from build123d import *

# Parameters (mm, degrees)
FILLET_4_R      = 3
F_4_0MM_4_D     = 4
F_4_0MM_4_DEPTH = 8
F_4_0MM_4_TIP   = 1.201721238
F_4_0MM_5_D     = 4
F_4_0MM_5_DEPTH = 7
F_4_0MM_5_TIP   = 1.201721238


# Read off the part's stored shape, not the designer's step: M16 机械螺纹 螺柱1
with BuildPart() as part:
    # 草图1 → 旋转1 (revolve)
    with BuildSketch(Plane.XY, mode=Mode.PRIVATE) as revolve_1_sk:
        Polygon((0, 0), (0, 8), (27, 8), (27, 8.5), (83, 8.5), (83, 18), (65, 18), (65, 27), (113, 27), (113, 18), (95, 18), (95, 8.5), (140, 8.5), (140, 0), align=None)
    revolve(revolve_1_sk.sketch.rotate(Axis((0, 0, 0), (1, 0, 0)), 90), axis=Axis((0, 0, 0), (1, 0, 0)))

    # 圆角4
    fillet_4_edges = [part.edges().sort_by_distance(p)[0] for p in [
        (95, 0, -8.5),
        (95, 0, -18),
        (83, 0, -18),
        (83, 0, -8.5),
    ]]
    fillet(fillet_4_edges, radius=FILLET_4_R)

    # M16 机械螺纹 螺柱1 outline → M16 机械螺纹 螺柱1 (revolve, cut)
    with BuildSketch(Plane.YX):
        Polygon((8, 1.0825), (6.9175, 0), (8, 0), align=None)
    revolve(axis=Axis((0, 0, 0), (1, 0, 0)), mode=Mode.SUBTRACT)

    # Ø4.0mm 暗销孔4
    with Locations(Plane(origin=(17.1, 8, 0), x_dir=(0, 0, 1), z_dir=(0, 1, 0))):
        with Locations((0, 0)):
            Hole(F_4_0MM_4_D / 2, depth=F_4_0MM_4_DEPTH)
            with Locations((0, 0, -(F_4_0MM_4_DEPTH + F_4_0MM_4_TIP / 2))):  # 118° drill point
                Cone(0, F_4_0MM_4_D / 2, F_4_0MM_4_TIP, mode=Mode.SUBTRACT)

    # Ø4.0mm 暗销孔5
    with Locations(Plane(origin=(140, 0, 0), x_dir=(0, 0, -1), z_dir=(1, 0, 0))):
        with Locations((0, 0)):
            Hole(F_4_0MM_5_D / 2, depth=F_4_0MM_5_DEPTH)
            with Locations((0, 0, -(F_4_0MM_5_DEPTH + F_4_0MM_5_TIP / 2))):  # 118° drill point
                Cone(0, F_4_0MM_5_D / 2, F_4_0MM_5_TIP, mode=Mode.SUBTRACT)


solid = part.part
Here's how the part is built. I have some questions about the finished solid (model axes, mm). A direction names the side the tool comes from. Coordinates: 2 decimals unless noted, no trailing zeros. Write each loop counter-clockwise with the first axis right and the second up, starting at its lowest first coordinate (ties: lowest second). Pieces come first, ordered by that corner, then holes.
1) If we section it at D-D (y = 21): List the corners of the cut face in (x, z) for me.
Filled in:
outline: (65, -16.97) - (113, -16.97) - (113, 16.97) - (65, 16.97) - close
2) Thinking about a two-plate mould opening in Y: for faces 4 (the face through (119.294, -8.428, -1.107)), 5 (the face through (89.34, 26.36, -5.85)), 6 (the face through (15.148, 3.948, 0.434)), 7 (the face through (17.204, -0.993, 0.331)), which applies, +Y half, -Y half, draft (parallel to the pull), parting line (faces both ways), or undercut?
Filled in:
face 4: undercut
face 5: parting line
face 6: draft
face 7: +Y half
3) I'm going to push flat-ended pins straight in: pin 1 (12 mm diameter, centred on y = -3.5, z = -17.5, fed in from -X); pin 2 (8 mm diameter, centred on x = 91, z = -15.5, fed in from +Y); pin 3 (13.5 mm diameter, centred on y = 1.5, z = -3, fed in from -X); pin 4 (3 mm diameter, centred on y = 7.5, z = -13.5, fed in from -X). Where does each tip first touch, or does it pass through?
Filled in:
pin 1: stops at x = 65
pin 2: stops at y = 24.43
pin 3: stops at x = 0
pin 4: stops at x = 82.29
4) If we section it at A-A (x = 102): List the corners of the cut face in (y, z) for me, plus the area to 3 significant figures.
Filled in:
outline: circle Ø54 at (0, 0); circle Ø17 at (0, 0); hole circle Ø36 at (0, 0)
area: 1,500 mm2
5) Which directions (+Z, -Z, +X, -X, +Y, -Y) give clear straight access to the entire face, cutting with the end or side of a thin tool? Please do faces 1 (the face through (113, 18, 6)), 2 (the face through (0, 0, 0)), 3 (the face through (72.395, -12.165, -13.267)).
Filled in:
face 1: +X
face 2: +Z, -Z, -X, +Y, -Y
face 3: -X
6) If we section it at C-C (z = -23): List the corners of the cut face in (x, y) for me, plus the area to 3 significant figures.
Filled in:
outline: (65, -14.14) - (113, -14.14) - (113, 14.14) - (65, 14.14) - close
area: 1,360 mm2
7) If I drill on line 1 (Y direction, x = 74, z = 0); line 2 (X direction, y = 6, z = 0); line 3 (X direction, y = -20.5, z = 8), over which ranges is the centre line in solid material (lowest first)?
Filled in:
line 1: y = -27 to -18, -8.5 to 8.5, 18 to 27
line 2: x = 0 to 15.1, 19.1 to 140
line 3: x = 65 to 113
8) If we section it at B-B (x = 48): List the corners of the cut face in (y, z) for me, plus the area to 3 significant figures.
Filled in:
outline: circle Ø17 at (0, 0)
area: 227 mm2
